Source: CAD feature listing. Evaluate the final solid. Frame: model axes, mm. Give positions to 0.01 mm unless a question says otherwise; leave off trailing zeros. Order: outer loops, then holes, each group sorted by start corner. A loop starts at its lowest first (then second) coordinate and runs counter-clockwise, first axis right, second up. Notation, with made-up numbers: M 24,34.25 L 52,34.25 A24 cw 52,50.25 Z; hole C -33,-36.5 d2. An arc over 180 degrees is marked long. Answer in a Markdown table with one row per item. Add a question column.
(1) Section query C-C, the plane y = -221. Return loops of the section in (x, z).
(2) Pin query (flat end, axial travel): P1, Ø1.5, axis at x = -46.5, z = 353, coming from the -Y side; P2, Ø1.5, axis at y = -34, z = 251.5, coming from the +X side; P3, Ø10, axis at y = -240, z = 260.5, coming from the -X side. Return the tip coordinate at first contact, or that it passes through.
(3) Material intervals for line 1 along X through (y, z) = (-0.5, 265); line 2 along Y through (x, z) = (-46.55, 369); line 3 along Z through (x, y) = (-48.05, -341), sorted ascending.
(4) Mould query, pull axis Z, two halves, no side actions, for faces 1 (the face through (-47.072, 13.975, 401.658)), 2 (the face through (-47.072, -4.244, 365.739)), 3 (the face through (-47.065, -368.915, 169.701)). Classes: pulls with the +Z half, pulls with the -Z half, needs draft (parallel to the pull), parting line crosses it, or undercut.
(5) Section query B-B, the plane x = -45.85. Count the separate pieces of the cut face and the enclosed holes in it, plus the area to 3 significant figures.
(6) Section query A-A, the plane z = 331. Return loops of the section in (x, y).
from build123d import *

# Parameters (mm, degrees)
F1_DEPTH = 120
F2_R     = 6
F3_DEPTH = 5
F4_R     = 6
F5_DEPTH = 5


with BuildPart() as f1:
    # F0 (on Top) → F1 (new body)
    with BuildSketch(Plane.XY):
        with BuildLine():
            Line((120.464271, 36.765282), (-39.183099, 36.765282))
            ThreePointArc((-39.183099, 36.765282), (-50.372007, 32.173501), (-54.535729, 20.818346))
            Line((-54.535729, 20.818346), (-54.535729, -83.234718))
            Line((-54.535729, -83.234718), (-49.535177, -83.234718))
            Line((-49.535177, -83.234718), (-49.536819, 10.563834))
            Line((-49.536819, 10.563834), (-49.537028, 22.530258))
            ThreePointArc((-49.537028, 22.530258), (-46.279821, 29.181243), (-39.340395, 31.767623))
            Line((-39.340395, 31.767623), (-28.383342, 31.767623))
            Line((-28.383342, 31.767623), (120.464271, 31.767623))
            Line((120.464271, 31.767623), (120.464271, 36.765282))
        make_face()
    extrude(amount=F1_DEPTH)

    # F2 (on face) → F3 (cut)
    with BuildSketch(Plane(origin=(0, 36.765282, 0), x_dir=(-1, 0, 0), z_dir=(0, 1, 0))):
        with Locations((-70.464271, 60)):
            Circle(F2_R)
        with Locations((-20.464271, 60)):
            Circle(F2_R)
    extrude(amount=-F3_DEPTH, mode=Mode.SUBTRACT)


with BuildPart() as f5:
    # F4 (on face) → F5 (new body)
    with BuildSketch(Plane(origin=(-49.536634, -0.000867, 0), x_dir=(-1.8e-05, 1, 0), z_dir=(1, 1.8e-05, 0))):
        with BuildLine():
            Line((-347.468874, 160.679807), (-7.468874, 160.679807))
            ThreePointArc((-7.468874, 160.679807), (13.744329, 169.466604), (22.531126, 190.679807))
            Line((22.531126, 190.679807), (22.531126, 380.679807))
            ThreePointArc((22.531126, 380.679807), (13.744329, 401.893011), (-7.468874, 410.679807))
            Line((-7.468874, 410.679807), (-97.468874, 410.679807))
            ThreePointArc((-97.468874, 410.679807), (-118.682078, 401.893011), (-127.468874, 380.679807))
            Line((-127.468874, 380.679807), (-127.468874, 280.679807))
            ThreePointArc((-127.468874, 280.679807), (-133.326739, 266.537672), (-147.468874, 260.679807))
            Line((-147.468874, 260.679807), (-357.468874, 260.679807))
            ThreePointArc((-357.468874, 260.679807), (-371.61101, 254.821943), (-377.468874, 240.679807))
            Line((-377.468874, 240.679807), (-377.468874, 190.679807))
            ThreePointArc((-377.468874, 190.679807), (-368.682078, 169.466604), (-347.468874, 160.679807))
        make_face()
        with Locations((-87.468874, 360.679807)):
            Circle(F4_R, mode=Mode.SUBTRACT)
        with Locations((-7.468874, 360.679807)):
            Circle(F4_R, mode=Mode.SUBTRACT)
    extrude(amount=F5_DEPTH)


solid = f5.part
Values follow:
| question | item | result |
|---|---|---|
| 1 | outline | M -49.53,160.68 L -44.53,160.68 L -44.53,260.68 L -49.53,260.68 Z |
| 2 | P1 | stops at y = -127.47 |
| 2 | P2 | stops at x = -44.54 |
| 2 | P3 | stops at x = -49.53 |
| 3 | line 1 | x = -49.54 to -44.54 |
| 3 | line 2 | y = -127.47 to 22.53 |
| 3 | line 3 | z = 160.68 to 260.68 |
| 4 | face 1 | pulls with the +Z half |
| 4 | face 2 | undercut |
| 4 | face 3 | pulls with the -Z half |
| 5 | separate pieces | 1 |
| 5 | enclosed holes | 2 |
| 5 | area | 61,500 mm² |
| 6 | outline | M -49.54,22.53 L -49.53,-127.47 L -44.53,-127.47 L -44.54,22.53 Z |
